Source: CAD feature listing. Evaluate the final solid. Frame: model axes, mm. Give positions to 0.01 mm unless a question says otherwise; leave off trailing zeros. Order: outer loops, then holes, each group sorted by start corner. A loop starts at its lowest first (then second) coordinate and runs counter-clockwise, first axis right, second up. Notation, with made-up numbers: M -9.75,46 L 16.25,46 A30 ccw 16.25,77 Z; hole C 65,-22.5 d11. An arc over 180 degrees is marked long. Return JSON: item names as keys, results as strings.
from build123d import *

# Parameters (mm, degrees)
SKETCH_W  = 50
SKETCH_H  = 50
SKETCH_R  = 5
PAD_DEPTH = 10


with BuildPart() as part:
    # Sketch → Pad (new body)
    with BuildSketch(Plane.XY):
        Rectangle(SKETCH_W, SKETCH_H)
        with Locations((12.5, 12.5)):
            Circle(SKETCH_R, mode=Mode.SUBTRACT)
        with Locations((-12.5, 12.5)):
            Circle(SKETCH_R, mode=Mode.SUBTRACT)
        with Locations((-12.5, -12.5)):
            Circle(SKETCH_R, mode=Mode.SUBTRACT)
        with Locations((12.5, -12.5)):
            Circle(SKETCH_R, mode=Mode.SUBTRACT)
    pad = extrude(amount=PAD_DEPTH)

    # Mirrored: Pad across face of Pad
    add(pad.mirror(Plane(origin=(0, -25, 5), x_dir=(1, 0, 0), z_dir=(0, -1, 0))))


solid = part.part
1. Section query C-C (z = 1.75). State how many separate pieces and enclosed holes the cut face has, then the cut area to 3 significant figures.
Evaluation:
{"separate pieces": "1", "enclosed holes": "8", "area": "4,370 mm^2"}
2. Draft query along X for faces 1 (the face through (15.188, -66.716, 4.93)), 2 (the face through (0, -26, 10)), 3 (the face through (15.188, -41.716, 4.93)), 4 (the face through (-25, -24, 5)). Return one class per face: pulls with the +X half, pulls with the -X half, needs draft (parallel to the pull), parting line crosses it, or undercut.
Evaluation:
{"face 1": "undercut", "face 2": "needs draft", "face 3": "undercut", "face 4": "pulls with the -X half"}
3. First-contact query: pin 1 (8 mm diameter, centred on x = 12.5, y = -37.5, fed in from -Z). Flat tip, straight axial feed; report the tip coordinate or a pass-through.
Evaluation:
{"pin 1": "passes through"}
4. Section query A-A (y = -37.5). Return loops of the section in (x, z).
Evaluation:
{"outline": "M -25,0 L -17.5,0 L -17.5,10 L -25,10 Z; M -7.5,0 L 7.5,0 L 7.5,10 L -7.5,10 Z; M 17.5,0 L 25,0 L 25,10 L 17.5,10 Z"}
5. Section query D-D (y = -65.5). Return loops of the section in (x, z).
Evaluation:
{"outline": "M -25,0 L -16.5,0 L -16.5,10 L -25,10 Z; M -8.5,0 L 8.5,0 L 8.5,10 L -8.5,10 Z; M 16.5,0 L 25,0 L 25,10 L 16.5,10 Z"}
6. Section query B-B (x = 12.5). Return loops of the section in (y, z), then the cut area to 3 significant figures.
Evaluation:
{"outline": "M -75,0 L -67.5,0 L -67.5,10 L -75,10 Z; M -57.5,0 L -42.5,0 L -42.5,10 L -57.5,10 Z; M -32.5,0 L -17.5,0 L -17.5,10 L -32.5,10 Z; M -7.5,0 L 7.5,0 L 7.5,10 L -7.5,10 Z; M 17.5,0 L 25,0 L 25,10 L 17.5,10 Z", "area": "600 mm^2"}
7. Ray query, probe 1 along X at (y, z) = (-37.5, 4); probe 2 along Y at (x, z) = (-12.5, 4.5); probe 3 along X at (y, z) = (15.5, 9.25). Return the intervals inside material, ascending.
Evaluation:
{"probe 1": "x = -25 to -17.5, -7.5 to 7.5, 17.5 to 25", "probe 2": "y = -75 to -67.5, -57.5 to -42.5, -32.5 to -17.5, -7.5 to 7.5, 17.5 to 25", "probe 3": "x = -25 to -16.5, -8.5 to 8.5, 16.5 to 25"}
